from build123d import *

# Parameters (mm, degrees)
BOSS_EXTRUDE1_DEPTH     = 20
SKETCH2_W               = 38
SKETCH2_H               = 4
BOSS_EXTRUDE2_DEPTH     = 12
FILLET1_R               = 5
SKETCH3_W               = 38
SKETCH3_H               = 4
BOSS_EXTRUDE3_DEPTH     = 25
SKETCH4_R               = 3.5
SKETCH4_R_2             = 1.5
BOSS_EXTRUDE4_DEPTH     = 2
SKETCH5_R               = 1.5
CUT_EXTRUDE1_DEPTH      = 49.713447835
CUT_EXTRUDE2_DEPTH      = 10
CUT_EXTRUDE3_DEPTH      = 50.689032995
CUT_EXTRUDE3_DEPTH_BACK = 50.689032995
SKETCH7_R               = 1


with BuildPart() as part:
    # Sketch1 → Boss-Extrude1 (new body)
    with BuildSketch(Plane(origin=(0, 0, 0), x_dir=(1, 0, 0), z_dir=(0, 1, 0))):
        Polygon((0, 12), (0, 0), (38, 0), (38, 12), (35, 12), (35, 4), (1, 4), (1, 12), align=None)
    extrude(amount=BOSS_EXTRUDE1_DEPTH)

    # Sketch2 → Boss-Extrude2 (add)
    with BuildSketch(Plane.XZ):
        with Locations((19, -2)):
            Rectangle(SKETCH2_W, SKETCH2_H)
    extrude(amount=BOSS_EXTRUDE2_DEPTH)

    # Fillet1
    fillet1_edges = [part.edges().sort_by_distance(p)[0] for p in [
        (36.5, 0, -4),
        (0.5, 0, -4),
    ]]
    fillet(fillet1_edges, radius=FILLET1_R)

    # Sketch3 → Boss-Extrude3 (add)
    with BuildSketch(Plane.XY):
        with Locations((19, -10)):
            Rectangle(SKETCH3_W, SKETCH3_H)
    extrude(amount=BOSS_EXTRUDE3_DEPTH)

    # Sketch4 → Boss-Extrude4 (add)
    with BuildSketch(Plane.XY):
        with Locations(Location((15, -0.5, 0), (0, 0, 180))):
            Circle(SKETCH4_R)
        with Locations((15, -0.5)):
            Circle(SKETCH4_R_2, mode=Mode.SUBTRACT)
    extrude(amount=BOSS_EXTRUDE4_DEPTH)

    # Sketch5 → Cut-Extrude1 (cut, through all)
    with BuildSketch(Plane.XY.offset(2)):
        with Locations(Location((15, -0.5, 0), (0, 0, 180))):
            Circle(SKETCH5_R)
    extrude(amount=-CUT_EXTRUDE1_DEPTH, mode=Mode.SUBTRACT)

    # Sketch6 → Cut-Extrude2 (cut)
    with BuildSketch(Plane(origin=(0, -8, 0), x_dir=(1, 0, 0), z_dir=(0, 1, 0))):
        Polygon((0, -25), (38, -4), (38, -25), align=None)
    extrude(amount=-CUT_EXTRUDE2_DEPTH, mode=Mode.SUBTRACT)

    # Sketch7 → Cut-Extrude3 (cut, two sides: drawn at the far end of the back side and taken through both)
    with BuildSketch(Plane.ZY.offset(-CUT_EXTRUDE3_DEPTH_BACK)):
        with Locations((-7, 15)):
            Circle(SKETCH7_R)
        with Locations((-7, 5)):
            Circle(SKETCH7_R)
    extrude(amount=CUT_EXTRUDE3_DEPTH + CUT_EXTRUDE3_DEPTH_BACK, mode=Mode.SUBTRACT)


solid = part.part
The listing builds one solid part. Answer for the finished solid, in the listing's coordinates (mm). A direction names the side the tool comes from. Coordinates: 2 decimals unless noted, no trailing zeros. Loops run counter-clockwise (first coordinate to the right, second up) from the corner with the lowest first, then second, coordinate; pieces in that order, holes last. Notation, with made-up numbers: (-34.75, -17.75) -> (19.25, -17.75) arc R30 ccw to (19.25, 8.25) -> close; hole circle Ø11 at (11, 16). An arc over 180 degrees is marked (long way). Write item = value, one per line. Start each with the question number.
1) A cutting plane is placed at B-B (x = 15). Give the vertices of the cut face in (y, z).
2) The mould has two halves that part along Y. Classify faces 5 (the face through (0.51, -1.43, -5.5)), 6 (the face through (18.73, -9.97, 14.65)), 7 (the face through (37, 14, -7)), 8 (the face through (11.66, -1.55, 0.99)): released by +Y, released by -Y, zero draft, split by the parting line, or undercut.
3) A cutting plane is placed at D-D (x = 9.5). Give the vertices of the cut face in (y, z), then the cut area to 3 significant figures.
4) A cutting plane is placed at C-C (z = -7). Give the vertices of the cut face in (x, y).
5) A cutting plane is placed at A-A (y = 15). Give the vertices of the cut face in (x, z).
6) Given pin 1 Ø8 at (x, y) = (16.5, 4) entering from -Z; pin 2 Ø5 at (x, y) = (30.5, 15.5) entering from +Z; pin 3 Ø2.5 at (x, z) = (36, -11) entering from -Y, each flat-ended and moving along its own axis, determine where each tip first touches the part or whether it passes through.
7) Straight lines are drawn through the part: line 1 (Y direction, x = 36.7, z = -7); line 2 (Z direction, x = 35.6, y = 5); line 3 (X direction, y = 8, z = -8). For each, find the intervals that lie inside material, in ascending order. Write a range as from..to.
8) A tool of negligible diameter and unlimited length cuts with its end or side. For faces 1 (the face through (13, -1, 2)), 2 (the face through (36, 0, -11)), 3 (the face through (15, -12, 7)), 4 (the face through (1, 10, -8)), from which of +Z, -Z, +X, -X, +Y, -Y can it reach the whole face along a straight path? Write none if from no direction.
Responses:
q1.outline = (-12, -4) -> (-2, -4) -> (-2, 2) -> (-4, 2) -> (-4, 0) -> (-8, 0) -> (-8, 16.71) -> (-12, 16.71) -> close; (1, -4) -> (20, -4) -> (20, 0) -> (3, 0) -> (3, 2) -> (1, 2) -> close
q2.face_5 = released by -Y
q2.face_6 = zero draft
q2.face_7 = undercut
q2.face_8 = undercut
q3.outline = (-12, -4) -> (20, -4) -> (20, 0) -> (-8, 0) -> (-8, 19.75) -> (-12, 19.75) -> close
q3.area = 207 mm²
q4.outline = (0, -0.42) -> (1, -0.42) -> (1, 4) -> (0, 4) -> close; (0, 6) -> (1, 6) -> (1, 14) -> (0, 14) -> close; (0, 16) -> (1, 16) -> (1, 20) -> (0, 20) -> close; (35, -0.42) -> (38, -0.42) -> (38, 4) -> (35, 4) -> close; (35, 6) -> (38, 6) -> (38, 14) -> (35, 14) -> close; (35, 16) -> (38, 16) -> (38, 20) -> (35, 20) -> close
q5.outline = (0, -12) -> (1, -12) -> (1, -8) -> (0, -8) -> close; (0, -6) -> (1, -6) -> (1, -4) -> (35, -4) -> (35, -6) -> (38, -6) -> (38, 0) -> (0, 0) -> close; (35, -12) -> (38, -12) -> (38, -8) -> (35, -8) -> close
q6.pin_1 = -4
q6.pin_2 = 0
q6.pin_3 = 0
q7.line_1 = -0.42..4, 6..14, 16..20
q7.line_2 = -12..-8, -6..0
q7.line_3 = 0..1, 35..38
q8.face_1 = +Z, +X, -X, +Y
q8.face_2 = -Z, +X, -X, -Y
q8.face_3 = +Z, -Z, +X, -X, -Y
q8.face_4 = -Z, +Y, -Y
